Geometry check sheet. Reference: the model listing, model coordinates, mm. Give positions to 0.01 mm unless a question says otherwise; leave off trailing zeros. Write each loop counter-clockwise with the first axis right and the second up, starting at its lowest first coordinate (ties: lowest second). Pieces come first, ordered by that corner, then holes. Notation, with made-up numbers: M 85,22.5 L 108,22.5 A19 ccw 108,30.5 Z; hole C 78,42.5 d6. An arc over 180 degrees is marked long. Use one line per item in the form item = value. Start each with the question number.
Autodesk Inventor part; units mm, degrees
ref_plane "YZ Plane" through (0, 0, 0) normal (1, 0, 0) x (0, 1, 0)
ref_plane "XZ Plane" through (0, 0, 0) normal (0, 1, 0) x (-1, 0, 0)
ref_plane "XY Plane" through (0, 0, 0) normal (0, 0, 1) x (1, 0, 0)
sketch "Sketch1" plane through (0, 0, 0) normal (0, 1, 0) x (-1, 0, 0)
  circle A0 centre (0, 0) radius 109.5
  circle A1 centre (0, 0) radius 62.5
  circle A2 centre (0, 0) radius 65
  dimension "d0" = 219
  dimension "d1" = 125
  dimension "d2" = 130
extrude "Extrusion1" add sketch "Sketch1" along normal blind 5 contours A0 | A2
extrude "Extrusion2" cut sketch "Sketch1" along normal blind 2.55 contours A2
sketch "Sketch2" plane through (0, 0, 0) normal (0, -1, 0) x (1, 0, 0)
  circle A0 centre (0, 0) radius 75
  circle A1 centre (0, 0) radius 76
  dimension "d7" = 150
  dimension "d8" = 152
extrude "Extrusion3" cut sketch "Sketch2" against normal blind 0.5
sketch "Sketch3" plane through (0, 5, 0) normal (0, 1, 0) x (1, 0, 0)
  circle A0 centre (0, 0) radius 82.5
  dimension "d11" = 165
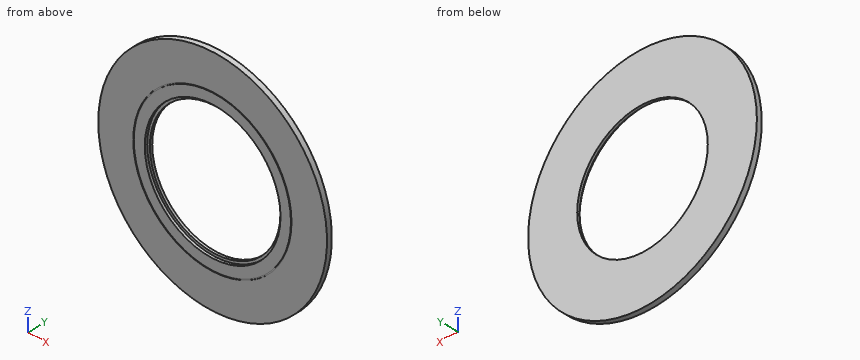
(1) Sectioned sample at B-B, the plane z = 0. Record the boundary of the cut face in (x, y), plus the area to 3 significant figures.
(2) Sectioned sample at C-C, the plane y = 3.9. Record the boundary of the cut face in (x, z), plus the area to 3 significant figures.
(3) Thickness scan on probe 1 along Z at (x, y) = (0, 0.3); probe 2 along X at (y, z) = (0.2, 57.5); probe 3 along X at (y, z) = (0.75, 20). Record the ranges inside material, lowest first. Write a range as [from, to].
(4) Sectioned sample at D-D, the plane x = -68. Record the boundary of the cut face in (y, z), plus the area to 3 significant figures.
(5) Depth check by flat-ended pin: pin 1 (1.5 mm diameter, centred on y = 2.5, z = -74, fed in from -X). Enter the tip coordinate at first touch or a pass-through.
(6) Sectioned sample at A-A, the plane x = 0. Record the boundary of the cut face in (y, z), plus the area to 3 significant figures.
Numbers:
q1.outline = M -109.5,0 L -76,0 L -76,0.5 L -75,0.5 L -75,0 L -65,0 L -65,2.55 L -62.5,2.55 L -62.5,5 L -109.5,5 Z; M 62.5,2.55 L 65,2.55 L 65,0 L 75,0 L 75,0.5 L 76,0.5 L 76,0 L 109.5,0 L 109.5,5 L 62.5,5 Z
q1.area = 456 mm2
q2.outline = C 0,0 d219; hole C 0,0 d125
q2.area = 25,400 mm2
q3.probe_1 = [-109.5, -76], [-75, -65], [65, 75], [76, 109.5]
q3.probe_2 = [-93.19, -49.7], [-48.15, -30.31], [30.31, 48.15], [49.7, 93.19]
q3.probe_3 = [-107.66, -61.85], [61.85, 107.66]
q4.outline = M 0,-85.83 L 5,-85.83 L 5,85.83 L 0,85.83 L 0,33.94 L 0.5,33.94 L 0.5,31.64 L 0,31.64 L 0,-31.64 L 0.5,-31.64 L 0.5,-33.94 L 0,-33.94 Z
q4.area = 856 mm2
q5.pin_1 = -81.39
q6.outline = M 0,-109.5 L 5,-109.5 L 5,-62.5 L 2.55,-62.5 L 2.55,-65 L 0,-65 L 0,-75 L 0.5,-75 L 0.5,-76 L 0,-76 Z; M 0,65 L 2.55,65 L 2.55,62.5 L 5,62.5 L 5,109.5 L 0,109.5 L 0,76 L 0.5,76 L 0.5,75 L 0,75 Z
q6.area = 456 mm2
